from build123d import *

# Parameters (mm, degrees)
EXTRUDE1_DEPTH  = 3.175
SKETCH2_W       = 3.175
SKETCH2_H       = 12.7
EXTRUDE2_DEPTH  = 3.175
LPATTERN1_COUNT = 3
LPATTERN1_PITCH = 50.8


with BuildPart() as part:
    # Sketch1 → Extrude1 (new body)
    with BuildSketch(Plane.XY):
        Polygon((0, 0), (50.8, 0), (50.8, 116.397422652), align=None)
    extrude(amount=EXTRUDE1_DEPTH)

    # Sketch2 → Extrude2 (add)
    with BuildSketch(Plane(origin=(0, 0, 0), x_dir=(0, 0, 1), z_dir=(-0.916515139, 0.4, 0))):
        with Locations((1.5875, 6.35)):
            Rectangle(SKETCH2_W, SKETCH2_H)
    extrude2 = extrude(amount=EXTRUDE2_DEPTH)

    # LPattern1: Extrude2 ×3
    with Locations(*[Vector(0.4, 0.916515139, 0) * (i * LPATTERN1_PITCH) for i in range(1, LPATTERN1_COUNT)]):
        add(extrude2)


solid = part.part
Source: CAD feature listing. Evaluate the final solid. Frame: model axes, mm. A direction names the side the tool comes from. Coordinates: 2 decimals unless noted, no trailing zeros. Write each loop counter-clockwise with the first axis right and the second up, starting at its lowest first coordinate (ties: lowest second). Pieces come first, ordered by that corner, then holes. Notation, with made-up numbers: M 24.5,69.5 L 81.5,69.5 A23 cw 81.5,101.5 Z; hole C -34,12 d11. An arc over 180 degrees is marked long. Use a Markdown table: item, result.
1) Section D-D, the plane x = 13. Output: boundary loops of the cut face in (y, z) (3 decimals).
Conclusion:
| item | result |
|---|---|
| outline | M 0,0 L 29.787,0 L 29.787,3.175 L 0,3.175 Z |
2) Ray query, L1, parallel to X at y = 74, z = 2.9; L2, parallel to X at y = 38, z = 2.35; L3, parallel to Y at x = 8, z = 0.75. Return the intervals inside material, ascending.
Conclusion:
| item | result |
|---|---|
| L1 | x = 32.3 to 50.8 |
| L2 | x = 16.58 to 50.8 |
| L3 | y = 0 to 18.33 |
3) Section A-A, the plane z = 2.35. Output: boundary loops of the cut face in (x, y).
Conclusion:
| item | result |
|---|---|
| outline | M -2.91,1.27 L 0,0 L 50.8,0 L 50.8,116.4 L 45.72,104.76 L 42.81,106.03 L 37.73,94.39 L 40.64,93.12 L 25.4,58.2 L 22.49,59.47 L 17.41,47.83 L 20.32,46.56 L 5.08,11.64 L 2.17,12.91 Z |
4) Reachability of faces 1 (the flat face through (50.8, 57, 2)), 2 (the flat face through (18.885, 47.185, 1.565)), 3 (the flat face through (23.965, 58.825, 1.565)) from +Z, -Z, +X, -X, +Y, -Y: full face, straight path, thin tool, end or side. Return the list, or none.
Conclusion:
| item | result |
|---|---|
| face 1 | +Z, -Z, +X, +Y, -Y |
| face 2 | +Z, -Z, -X |
| face 3 | +Z, -Z, +Y |
5) Section B-B, the plane x = 39. Output: boundary loops of the cut face in (y, z) (3 decimals), then the cut area to 3 significant figures.
Conclusion:
| item | result |
|---|---|
| outline | M 0,0 L 89.36,0 L 89.36,3.175 L 0,3.175 Z; M 93.834,0 L 97.298,0 L 97.298,3.175 L 93.834,3.175 Z |
| area | 295 mm^2 |
6) Mould query, pull axis Y, two halves, no side actions, for faces 4 (the flat face through (-1.435, 0.626, 1.565)), 5 (the flat face through (40.306, 100.289, 1.565)), 6 (the flat face through (12.807, 29.344, 1.565)). Classes: pulls with the +Y half, pulls with the -Y half, needs draft (parallel to the pull), parting line crosses it, or undercut.
Conclusion:
| item | result |
|---|---|
| face 4 | pulls with the -Y half |
| face 5 | pulls with the +Y half |
| face 6 | undercut |
7) Section C-C, the plane y = 67. Output: boundary loops of the cut face in (x, z) (3 decimals), then the cut area to 3 significant figures.
Conclusion:
| item | result |
|---|---|
| outline | M 29.241,0 L 50.8,0 L 50.8,3.175 L 29.241,3.175 Z |
| area | 68.4 mm^2 |
